Design review of the part built by this model. Coordinates are the model's own, in mm. Round coordinates to 2 decimals unless told otherwise and drop trailing zeros. Order: outer loops, then holes, each group sorted by start corner. A loop starts at its lowest first (then second) coordinate and runs counter-clockwise, first axis right, second up. Notation, with made-up numbers: M -23,85 L 20,85 A35 cw 20,123 Z; hole C 67.5,-11 d1. An arc over 180 degrees is marked long. Write item = value, one per line. Start each with the question number.
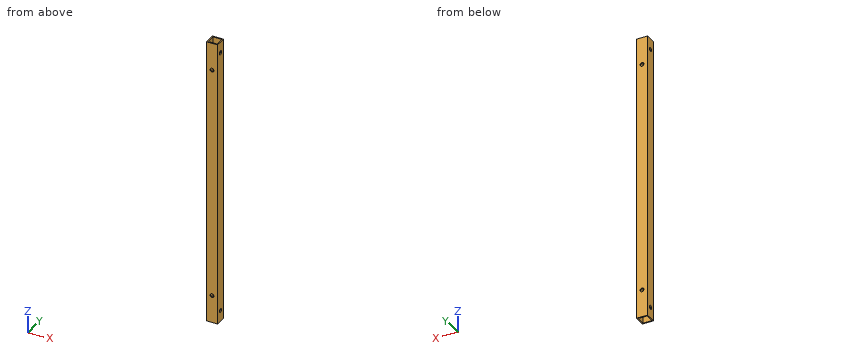
Autodesk Inventor part; units mm, degrees
ref_plane "YZ Plane" through (0, 0, 0) normal (1, 0, 0) x (0, 1, 0)
ref_plane "XZ Plane" through (0, 0, 0) normal (0, 1, 0) x (-1, 0, 0)
ref_plane "XY Plane" through (0, 0, 0) normal (0, 0, 1) x (1, 0, 0)
sketch "スケッチ1" plane through (0, 0, 0) normal (0, 0, 1) x (1, 0, 0)
  line L0 (5, -5) -> (-5, -5)
  line L1 (-5, -5) -> (-5, 5)
  line L2 (-5, 5) -> (5, 5)
  line L3 (5, 5) -> (5, -5)
  line L4 (5, -5) -> (-5, 5) construction
  line L5 (-5, -5) -> (5, 5) construction
  line L6 (4, 4) -> (-4, 4)
  line L7 (-4, 4) -> (-4, -4)
  line L8 (-4, -4) -> (4, -4)
  line L9 (4, -4) -> (4, 4)
  point P0 (0, 0)
  dimension "d0" = 10
  dimension "d1" = 10
  dimension "d2" = 1
extrude "押し出し1" add sketch "スケッチ1" along normal blind 260
sketch "スケッチ2" plane through (5, -5, 0) normal (1, 0, 0) x (0, 0, -1)
  line L0 (0, 5) -> (-228.6606, 5)
  line L1 (0, 0) -> (0, 10)
  point P0 (-250, 5)
  point P1 (-10, 5)
  dimension "d5" = 240
  dimension "d6" = 10
hole "穴1" at (5, 0, 250) at (5, 0, 10) direction (-1, 0, 0) diameter 3.5 end through all
sketch "スケッチ3" plane through (-5, 5, 0) normal (0, 1, 0) x (1, 0, 0)
  line L0 (5, 0) -> (5, -260)
  line L1 (9, -260) -> (1, -260)
  line L2 (10, 0) -> (0, 0)
  point P0 (5, -235)
  point P1 (5, -25)
  dimension "d14" = 25
  dimension "d23" = 25
hole "穴2" at (0, 5, 235) at (0, 5, 25) direction (0, -1, 0) diameter 3.5 end through all
properties part number "small_kaku_1010_bridge_1020"
(1) Consider section A-A, the plane y = 0. Write out the cut boundary in (x, z).
(2) For line 1 along Z through (x, y) = (0, -4.6); line 2 along X through (y, z) = (2, 132); line 3 along Y through (x, z) = (-4.5, 10), list the stretches that pass through material, from the lowest coordinate up. Write a range as [from, to].
(3) Consider section B-B, the plane z = 164. Write out the cut boundary in (x, y).
(4) Insertion check: pin 1 (5 mm diameter, centred on x = -1.5, y = 3, fed in from -Z). The pin has a flat end and moves straight along its axis. Give the tip position at first contact, or say it passes through.
(5) Consider section C-C, the plane x = 0. Write out the cut boundary in (y, z), then the cut area to 3 significant figures.
Completed:
q1.outline = M -5,0 L -4,0 L -4,8.25 L -5,8.25 Z; M -5,11.75 L -4,11.75 L -4,248.25 L -5,248.25 Z; M -5,251.75 L -4,251.75 L -4,260 L -5,260 Z; M 4,0 L 5,0 L 5,8.25 L 4,8.25 Z; M 4,11.75 L 5,11.75 L 5,248.25 L 4,248.25 Z; M 4,251.75 L 5,251.75 L 5,260 L 4,260 Z
q2.line_1 = [0, 23.25], [26.75, 233.25], [236.75, 260]
q2.line_2 = [-5, -4], [4, 5]
q2.line_3 = [-5, -1.75], [1.75, 5]
q3.outline = M -5,-5 L 5,-5 L 5,5 L -5,5 Z; hole M -4,-4 L 4,-4 L 4,4 L -4,4 Z
q4.pin_1 = 0
q5.outline = M -5,0 L -4,0 L -4,23.25 L -5,23.25 Z; M -5,26.75 L -4,26.75 L -4,233.25 L -5,233.25 Z; M -5,236.75 L -4,236.75 L -4,260 L -5,260 Z; M 4,0 L 5,0 L 5,23.25 L 4,23.25 Z; M 4,26.75 L 5,26.75 L 5,233.25 L 4,233.25 Z; M 4,236.75 L 5,236.75 L 5,260 L 4,260 Z
q5.area = 506 mm2
